from build123d import *

# Parameters (mm, degrees)
SKETCH1_W           = 69.6
SKETCH1_H           = 49.1
BOSS_EXTRUDE1_DEPTH = 1.6
SKETCH2_R           = 9
BOSS_EXTRUDE2_DEPTH = 25
SKETCH3_R           = 1.55
CUT_EXTRUDE1_DEPTH  = 2.6
SKETCH4_W           = 7.135274134
SKETCH4_H           = 3.634808115
SKETCH4_W_2         = 8.411757442
SKETCH4_H_2         = 3.336029474
SKETCH4_W_3         = 8.448874517
SKETCH4_H_3         = 3.933927867
SKETCH4_W_4         = 5.945259598
SKETCH4_H_4         = 10.026659932
BOSS_EXTRUDE3_DEPTH = 5


with BuildPart() as part:
    # Sketch1 → Boss-Extrude1 (new body)
    with BuildSketch(Plane(origin=(0, 0, 0), x_dir=(1, 0, 0), z_dir=(0, 1, 0))):
        with Locations((34.8, -24.55)):
            Rectangle(SKETCH1_W, SKETCH1_H)
    extrude(amount=BOSS_EXTRUDE1_DEPTH)

    # Sketch2 → Boss-Extrude2 (add)
    with BuildSketch(Plane(origin=(0, 1.6, 0), x_dir=(1, 0, 0), z_dir=(0, 1, 0))):
        with Locations((17.528795591, -31.108165605)):
            Circle(SKETCH2_R)
        with Locations((28.327813128, -15.884294945)):
            Circle(SKETCH2_R)
        with Locations((43.352916856, -31.108165605)):
            Circle(SKETCH2_R)
    extrude(amount=BOSS_EXTRUDE2_DEPTH)

    # Sketch3 → Cut-Extrude1 (cut, through all)
    with BuildSketch(Plane(origin=(0, 1.6, 0), x_dir=(1, 0, 0), z_dir=(0, 1, 0))):
        with Locations((3.937, -4.318)):
            Circle(SKETCH3_R)
        with Locations((66.17, -4.29)):
            Circle(SKETCH3_R)
        with Locations((66.044, -45.29)):
            Circle(SKETCH3_R)
        with Locations((3.937, -45.29)):
            Circle(SKETCH3_R)
    extrude(amount=-CUT_EXTRUDE1_DEPTH, mode=Mode.SUBTRACT)

    # Sketch4 → Boss-Extrude3 (add)
    with BuildSketch(Plane(origin=(0, 1.6, 0), x_dir=(1, 0, 0), z_dir=(0, 1, 0))):
        with Locations((17.346192507, -1.817404058)):
            Rectangle(SKETCH4_W, SKETCH4_H)
        with Locations((52.850279958, -1.668014737)):
            Rectangle(SKETCH4_W_2, SKETCH4_H_2)
        with Locations((16.192473292, -47.133036066)):
            Rectangle(SKETCH4_W_3, SKETCH4_H_3)
        with Locations((57.291981259, -44.086670034)):
            Rectangle(SKETCH4_W_4, SKETCH4_H_4)
    extrude(amount=BOSS_EXTRUDE3_DEPTH)


solid = part.part
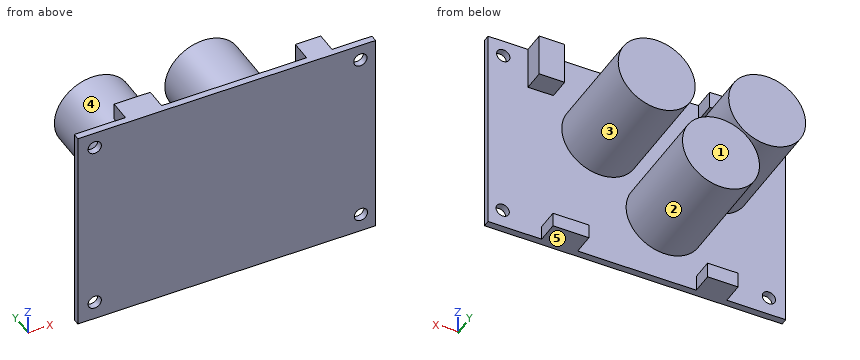
Model file for the job. Use its own axes, mm. Face numbers are marked on the shaded views. A direction names the side the tool comes from. Give positions to 0.01 mm unless a question says otherwise; leave off trailing zeros. Write each loop counter-clockwise with the first axis right and the second up, starting at its lowest first coordinate (ties: lowest second). Pieces come first, ordered by that corner, then holes. Notation, with made-up numbers: (-28.75, 84.25) - (-11.75, 84.25) arc R28 ccw to (-11.75, 103.25) - close; hole circle Ø10 at (-8, 11). An arc over 180 degrees is marked (long way). Answer as CSV lines item,"result".
1. Band-saw the part on D-D (y = 24). Write the cut outline in (x, z).
Responses:
outline,"circle Ø18 at (17.53, 31.11); circle Ø18 at (28.33, 15.88); circle Ø18 at (43.35, 31.11)"
2. Band-saw the part on A-A (x = 41). Write the cut outline in (y, z).
Responses:
outline,"(0, 0) - (1.6, 0) - (1.6, 22.42) - (26.6, 22.42) - (26.6, 39.8) - (1.6, 39.8) - (1.6, 49.1) - (0, 49.1) - close"
3. Two-plate mould, pull along X, no slides. Class the marked faces 1, 2 and 3: +X half, -X half, draft (parallel to the pull), parting line (faces both ways), or undercut.
Responses:
face 1,"draft"
face 2,"undercut"
face 3,"undercut"
4. Band-saw the part on B-B (z = 8). Write the cut outline in (x, y), and give its area (3 significant figures).
Responses:
outline,"(0, 0) - (69.6, 0) - (69.6, 1.6) - (32.67, 1.6) - (32.67, 26.6) - (23.99, 26.6) - (23.99, 1.6) - (0, 1.6) - close"
area,"328 mm2"
5. Band-saw the part on C-C (x = 66.17). Write the cut outline in (y, z), and give its area (3 significant figures).
Responses:
outline,"(0, 0) - (1.6, 0) - (1.6, 2.74) - (0, 2.74) - close; (0, 5.84) - (1.6, 5.84) - (1.6, 43.75) - (0, 43.75) - close; (0, 46.83) - (1.6, 46.83) - (1.6, 49.1) - (0, 49.1) - close"
area,"68.7 mm2"
6. Pin check, flat tips, straight feed: pin 1 (2.5 mm diameter, centred on x = 3.937, z = 45.29, fed in from -Y); pin 2 (3 mm diameter, centred on x = 29, y = 22.5, fed in from -Z); pin 3 (1 mm diameter, centred on y = 5, z = 2, fed in from +X); pin 4 (4 mm diameter, centred on y = 7, z = 22, fed in from +X). Stop position of each tip, or through.
Responses:
pin 1,"passes through"
pin 2,"stops at z = 6.88"
pin 3,"stops at x = 57.06"
pin 4,"stops at x = 48.87"
7. Drill centre lines: L1, parallel to X at y = 0.95, z = 4.29; L2, parallel to X at y = 1.25, z = 45.29; L3, parallel to Z at x = 66.17, y = 0.8. Where is each one in solid material? Low to high. Write a range as [from, to].
Responses:
L1,"x = [0, 2.39], [5.49, 64.62], [67.72, 69.6]"
L2,"x = [0, 2.39], [5.49, 64.49], [67.59, 69.6]"
L3,"z = [0, 2.74], [5.84, 43.75], [46.83, 49.1]"
8. 3-axis set-ups, long thin cutter, end or side, ignore diameter. For the marked faces 4 and 5: which of +Z, -Z, +X, -X, +Y, -Y reach the whole face in a straight line?
Responses:
face 4,"+Y"
face 5,"-Z, +X, -X, +Y, -Y"
